```python
from build123d import *

# Parameters (mm, degrees)
F0_R     = 3.5
F1_DEPTH = 12.5
F2_W     = 2
F2_H     = 9
F3_DEPTH = 3.75
F7_SIZE  = 2


with BuildPart() as f1:
    # F0 (on Top) → F1 (new body, symmetric)
    with BuildSketch(Plane.XY):
        Circle(F0_R)
    extrude(amount=F1_DEPTH, both=True)

    # F2 (on face) → F3 (join, symmetric)
    with BuildSketch(Plane(origin=(0, 0, -12.5), x_dir=(1, 0, 0), z_dir=(0, 0, -1))):
        Rectangle(F2_W, F2_H)
    extrude(amount=F3_DEPTH, both=True)

    # F5 (on face) → F6 (revolve)
    with BuildSketch(Plane.XY.offset(12.5)):
        with BuildLine():
            Line((4.5, 0), (-4.5, 0))
            ThreePointArc((-4.5, 0), (0, -4.5), (4.5, 0))
        make_face()
    revolve(axis=Axis((-0.09783, 0, 12.5), (1, 0, 0)))

    # F7
    f7_edges = [f1.edges().sort_by_distance(p)[0] for p in [
        (0, -4.5, -16.25),
        (0, 4.5, -16.25),
    ]]
    chamfer(f7_edges, length=F7_SIZE)


solid = f1.part
```
Work out the finished part from the listing and answer in its coordinate system (mm). A direction names the side the tool comes from. Give positions to 0.01 mm unless a question says otherwise; leave off trailing zeros. Order: outer loops, then holes, each group sorted by start corner. A loop starts at its lowest first (then second) coordinate and runs counter-clockwise, first axis right, second up.
1. Section B-B, the plane z = -10 is taken. Determine the outline of the cut face in (x, y).
Result sheet:
outline: (-1, -4.5) - (1, -4.5) - (1, -3.35) arc R3.5 ccw to (1, 3.35) - (1, 4.5) - (-1, 4.5) - (-1, 3.35) arc R3.5 ccw to (-1, -3.35) - close
2. Section C-C, the plane x = 0 is taken. Determine the outline of the cut face in (y, z).
Result sheet:
outline: (-4.5, -14.25) - (-2.5, -16.25) - (2.5, -16.25) - (4.5, -14.25) - (4.5, -8.75) - (3.5, -8.75) - (3.5, 9.67) arc R4.5 ccw (long way) to (-3.5, 9.67) - (-3.5, -8.75) - (-4.5, -8.75) - close
3. Straight lines are drawn through the part: L1, parallel to Y at x = 0, z = 0.5; L2, parallel to X at y = 0.5, z = -14; L3, parallel to Z at x = 0.75, y = 4. For each, find the intervals that lie inside material, in ascending order.
Result sheet:
L1: y = -3.5 to 3.5
L2: x = -1 to 1
L3: z = -14.75 to -8.75, 10.58 to 14.42
4. The mould has two halves that part along Z. Classify faces 4 (the flat face through (0, 0, -16.25)), 5 (the flat face through (1, 0, -13)), 6 (the cylindrical face through (3.233, -1.341, -1.259)), 7 (the flat face through (0, 4, -8.75)): released by +Z, released by -Z, zero draft, split by the parting line, or undercut.
Result sheet:
face 4: released by -Z
face 5: zero draft
face 6: undercut
face 7: undercut
5. Each of these flat-tipped pins is pushed along its axis until it touches: P1, Ø1.5, axis at y = -1.5, z = -12.5, coming from the -X side; P2, Ø0.6, axis at x = 0, y = -4, coming from the +Z side; P3, Ø2, axis at y = -2, z = -0.5, coming from the +X side. Where does it stop, or does it pass through?
Result sheet:
P1: stops at x = -3.42
P2: stops at z = 15.06
P3: stops at x = 3.35
6. Section D-D, the plane z = -2 is taken. Determine the outline of the cut face in (x, y).
Result sheet:
outline: circle Ø7 at (0, 0)
7. For faces 1 (the flat face through (2, 0, -12.5)), 2 (the flat face through (0, 4.5, -12)), 3 (the flat face through (-2, 0, -12.5)), determine the directions among +Z, -Z, +X, -X, +Y, -Y from which every point of the face is accessible in a straight line to the end or side of a thin tool.
Result sheet:
face 1: -Z, +X, +Y, -Y
face 2: +Z, -Z, +X, -X, +Y
face 3: -Z, -X, +Y, -Y
8. Section A-A, the plane y = 0 is taken. Determine the outline of the cut face in (x, z).
Result sheet:
outline: (-3.5, -12.5) - (-1, -12.5) - (-1, -16.25) - (1, -16.25) - (1, -12.5) - (3.5, -12.5) - (3.5, 9.67) arc R4.5 ccw (long way) to (-3.5, 9.67) - close
